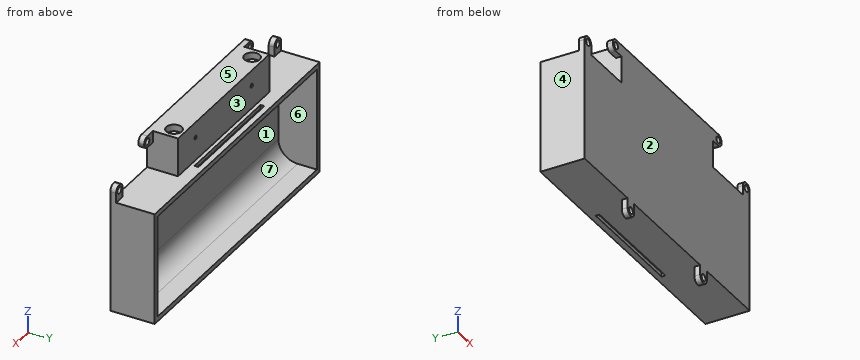
from build123d import *

# Parameters (mm, degrees)
SKETCH_1_W          = 83
SKETCH_1_H          = 20
EXTRUDE_1_DEPTH     = 16
SKETCH_2_R          = 4
CUT_EXTRUDE_1_DEPTH = 3.5
SKETCH_3_R          = 1
CUT_EXTRUDE_2_DEPTH = 10
SKETCH_6_R          = 1
CUT_EXTRUDE_5_DEPTH = 8
SKETCH_7_W          = 150
SKETCH_7_H          = 3
EXTRUDE_2_DEPTH     = 58
SKETCH_8_W          = 150
SKETCH_8_H          = 58
SKETCH_8_W_2        = 145
SKETCH_8_H_2        = 53
EXTRUDE_3_DEPTH     = 20
FILLET_1_R          = 10
CUT_EXTRUDE_START   = -45
SKETCH_9_W          = 2
SKETCH_9_H          = 2
CUT_EXTRUDE_6_DEPTH = 60
SKETCH_10_W         = 6
SKETCH_10_H         = 3
EXTRUDE_4_DEPTH     = 8
SKETCH_11_W         = 6
SKETCH_11_H         = 3
EXTRUDE_5_DEPTH     = 8
SKETCH_12_W         = 6
SKETCH_12_H         = 3
EXTRUDE_6_DEPTH     = 8
SKETCH_13_W         = 6
SKETCH_13_H         = 3
EXTRUDE_7_DEPTH     = 8
FILLET_2_R          = 3
SKETCH_14_R         = 1.75
CUT_EXTRUDE_7_DEPTH = 109.632407688


with BuildPart() as part:
    # 스케치1 → 보스-돌출1 (new body)
    with BuildSketch(Plane(origin=(0, 0, 0), x_dir=(1, 0, 0), z_dir=(0, 1, 0))):
        Rectangle(SKETCH_1_W, SKETCH_1_H)
    extrude(amount=EXTRUDE_1_DEPTH)

    # 스케치2 → 컷-돌출1 (cut)
    with BuildSketch(Plane.XY.offset(10)):
        with Locations((-35.5, 10.5)):
            Circle(SKETCH_2_R)
        with Locations((35.5, 10.5)):
            Circle(SKETCH_2_R)
    extrude(amount=-CUT_EXTRUDE_1_DEPTH, mode=Mode.SUBTRACT)

    # 스케치3 → 컷-돌출2 (cut)
    with BuildSketch(Plane(origin=(0, 16, 0), x_dir=(1, 0, 0), z_dir=(0, 1, 0))):
        with Locations(Location((-25.5, -2, 0), (0, 0, 270))):
            Circle(SKETCH_3_R)
        with Locations(Location((25.5, -2, 0), (0, 0, 270))):
            Circle(SKETCH_3_R)
    extrude(amount=-CUT_EXTRUDE_2_DEPTH, mode=Mode.SUBTRACT)

    # 스케치6 → 컷-돌출5 (cut)
    with BuildSketch(Plane.XY.offset(6.5)):
        with Locations((-35.5, 10.5)):
            Circle(SKETCH_6_R)
        with Locations((35.5, 10.5)):
            Circle(SKETCH_6_R)
    extrude(amount=-CUT_EXTRUDE_5_DEPTH, mode=Mode.SUBTRACT)

    # 스케치7 → 보스-돌출2 (add)
    with BuildSketch(Plane(origin=(0, 0, -10), x_dir=(-1, 0, 0), z_dir=(0, 0, -1))):
        with Locations((0, 1.5)):
            Rectangle(SKETCH_7_W, SKETCH_7_H)
    extrude(amount=EXTRUDE_2_DEPTH)

    # 스케치8 → 보스-돌출3 (add)
    with BuildSketch(Plane(origin=(0, 3, 0), x_dir=(1, 0, 0), z_dir=(0, 1, 0))):
        with Locations((0, 39)):
            Rectangle(SKETCH_8_W, SKETCH_8_H)
        with Locations((0, 39)):
            Rectangle(SKETCH_8_W_2, SKETCH_8_H_2, mode=Mode.SUBTRACT)
    extrude(amount=EXTRUDE_3_DEPTH)

    # 필렛1
    fillet_1_edges = [part.edges().sort_by_distance(p)[0] for p in [
        (0, 3, -65.5),
        (0, 3, -12.5),
    ]]
    fillet(fillet_1_edges, radius=FILLET_1_R)

    # 스케치9 → 컷-돌출6 (cut)
    with BuildSketch(Plane.ZY.offset(75).offset(CUT_EXTRUDE_START)):
        with Locations((-67, 19)):
            Rectangle(SKETCH_9_W, SKETCH_9_H)
        with Locations((-11, 19)):
            Rectangle(SKETCH_9_W, SKETCH_9_H)
    extrude(amount=-CUT_EXTRUDE_6_DEPTH, mode=Mode.SUBTRACT)

    # 스케치10 → 보스-돌출4 (add)
    with BuildSketch(Plane.XY.offset(-10)):
        with Locations((-72, 1.5)):
            Rectangle(SKETCH_10_W, SKETCH_10_H)
        with Locations((72, 1.5)):
            Rectangle(SKETCH_10_W, SKETCH_10_H)
    extrude(amount=EXTRUDE_4_DEPTH)

    # 스케치11 → 보스-돌출5 (add)
    with BuildSketch(Plane(origin=(0, 0, -68), x_dir=(-1, 0, 0), z_dir=(0, 0, -1))):
        with Locations((-33, 1.5)):
            Rectangle(SKETCH_11_W, SKETCH_11_H)
        with Locations((33, 1.5)):
            Rectangle(SKETCH_11_W, SKETCH_11_H)
    extrude(amount=EXTRUDE_5_DEPTH)

    # 스케치12 → 보스-돌출6 (add)
    with BuildSketch(Plane.ZY.offset(41.5)):
        with Locations((7, 1.5)):
            Rectangle(SKETCH_12_W, SKETCH_12_H)
    extrude(amount=EXTRUDE_6_DEPTH)

    # 스케치13 → 보스-돌출7 (add)
    with BuildSketch(Plane(origin=(41.5, 0, 0), x_dir=(0, 0, -1), z_dir=(1, 0, 0))):
        with Locations((-7, 1.5)):
            Rectangle(SKETCH_13_W, SKETCH_13_H)
    extrude(amount=EXTRUDE_7_DEPTH)

    # 필렛2
    fillet_2_edges = [part.edges().sort_by_distance(p)[0] for p in [
        (69, 1.5, -2),
        (75, 1.5, -2),
        (-75, 1.5, -2),
        (-69, 1.5, -2),
        (-36, 1.5, -76),
        (-30, 1.5, -76),
        (30, 1.5, -76),
        (36, 1.5, -76),
        (-49.5, 1.5, 4),
        (-49.5, 1.5, 10),
        (49.5, 1.5, 10),
        (49.5, 1.5, 4),
    ]]
    fillet(fillet_2_edges, radius=FILLET_2_R - 0.0001)  # a hair under: the kernel refuses the full size

    # 스케치14 → 컷-돌출7 (cut, through all)
    with BuildSketch(Plane(origin=(0, 3, 0), x_dir=(1, 0, 0), z_dir=(0, 1, 0))):
        with Locations(Location((-33, 73, 0), (0, 0, 270))):
            Circle(SKETCH_14_R)
        with Locations(Location((33, 73, 0), (0, 0, 270))):
            Circle(SKETCH_14_R)
        with Locations(Location((-46.5, -7, 0), (0, 0, 270))):
            Circle(SKETCH_14_R)
        with Locations(Location((46.5, -7, 0), (0, 0, 270))):
            Circle(SKETCH_14_R)
        with Locations(Location((72, 5, 0), (0, 0, 270))):
            Circle(SKETCH_14_R)
        with Locations(Location((-72, 5, 0), (0, 0, 270))):
            Circle(SKETCH_14_R)
    extrude(amount=-CUT_EXTRUDE_7_DEPTH, mode=Mode.SUBTRACT)


solid = part.part
The listing builds one solid part. Answer for the finished solid, in the listing's coordinates (mm). Face numbers are marked on the shaded views. A direction names the side the tool comes from. Coordinates: 2 decimals unless noted, no trailing zeros. Loops run counter-clockwise (first coordinate to the right, second up) from the corner with the lowest first, then second, coordinate; pieces in that order, holes last. Notation, with made-up numbers: (6.5, -5) -> (52.5, -5) arc R28 ccw to (52.5, 24) -> close; hole circle Ø5 at (75, 63). An arc over 180 degrees is marked (long way). Write item = value, one per line. Start each with the question number.
1) Straight lines are drawn through the part: line 1 (X direction, y = 1.4, z = 7); line 2 (X direction, y = 9.25, z = 2); line 3 (X direction, y = 2, z = -5). For each, find the intervals that lie inside material, in ascending order. Write a range as from..to.
2) A cutting plane is placed at A-A (x = 9). Give the vertices of the cut face in (y, z).
3) A tool of negligible diameter and unlimited length cuts with its end or side. For the marked faces 1, 2 and 3, from which of +Z, -Z, +X, -X, +Y, -Y can it reach the whole face along a straight path? Write none if from no direction.
4) Given pin 1 Ø1.6 at (x, y) = (-35.5, 10) entering from +Z; pin 2 Ø1 at (x, y) = (-43, 13) entering from -Z; pin 3 Ø3 at (x, z) = (-32.5, -71) entering from +Y, each flat-ended and moving along its own axis, determine where each tip first touches the part or whether it passes through.
5) A cutting plane is placed at B-B (z = -17). Give the vertices of the cut face in (x, y).
6) A cutting plane is placed at C-C (x = 57). Give the vertices of the cut face in (y, z).
7) The mould has two halves that part along Z. Classify the marked faces 4, 5, 6 and 7: released by +Z, released by -Z, zero draft, split by the parting line, or undercut.
Responses:
q1.line_1 = -49.5..-48.25, -44.75..44.75, 48.25..49.5
q1.line_2 = -41.5..-26.5, -24.5..24.5, 26.5..41.5
q1.line_3 = -75..-73.75, -70.25..-69, -41.5..41.5, 69..70.25, 73.75..75
q2.outline = (0, -68) -> (18, -68) -> (18, -66) -> (20, -66) -> (20, -68) -> (23, -68) -> (23, -65.5) -> (13, -65.5) arc R10 cw to (3, -55.5) -> (3, -22.5) arc R10 cw to (13, -12.5) -> (23, -12.5) -> (23, -10) -> (20, -10) -> (20, -12) -> (18, -12) -> (18, -10) -> (16, -10) -> (16, 10) -> (0, 10) -> close
q3.face_1 = +Y
q3.face_2 = +Z, -Z, +X, -X, -Y
q3.face_3 = +Z, +X, -X, +Y
q4.pin_1 = 6.5
q4.pin_2 = -68
q4.pin_3 = 3
q5.outline = (-75, 0) -> (75, 0) -> (75, 23) -> (72.5, 23) -> (72.5, 4.65) -> (-72.5, 4.65) -> (-72.5, 23) -> (-75, 23) -> close
q6.outline = (0, -68) -> (23, -68) -> (23, -65.5) -> (13, -65.5) arc R10 cw to (3, -55.5) -> (3, -22.5) arc R10 cw to (13, -12.5) -> (23, -12.5) -> (23, -10) -> (0, -10) -> close
q7.face_4 = zero draft
q7.face_5 = released by +Z
q7.face_6 = undercut
q7.face_7 = undercut
